```python
from build123d import *

# Parameters (mm, degrees)
F0_R     = 3.5687
F0_R_2   = 25.4
F1_DEPTH = 12.7
F2_R     = 25.39999
F3_R     = 19.05
F4_R     = 6.35


# Not quite as in the source:
# - a fillet or chamfer is up to 0.001 mm smaller than in the source, because OpenCascade refuses the exact size


with BuildPart() as f1:
    # F0 (on Top) → F1 (new body)
    with BuildSketch(Plane.XY):
        with BuildLine():
            Line((-25.4, -44.45), (0, -44.45))
            ThreePointArc((0, -44.45), (44.45, 0), (0, 44.45))
            Line((0, 44.45), (-25.4, 44.45))
            Line((-25.4, 44.45), (-25.4, 209.55))
            Line((-25.4, 209.55), (-138.1252, 322.2752))
            Line((-138.1252, 322.2752), (-352.425, 322.2752))
            Line((-352.425, 322.2752), (-352.425, 315.9252107143))
            Line((-352.425, 315.9252107143), (-387.35, 315.9252107143))
            Line((-387.35, 315.9252107143), (-387.35, 322.2752))
            Line((-387.35, 322.2752), (-584.2, 322.2752))
            Line((-584.2, 322.2752), (-584.2, 246.0752))
            Line((-584.2, 246.0752), (-187.648785695, 246.0752))
            Line((-187.648785695, 246.0752), (-114.3, 172.726414305))
            Line((-114.3, 172.726414305), (-114.3, -172.726414305))
            Line((-114.3, -172.726414305), (-200.348785695, -258.7752))
            Line((-200.348785695, -258.7752), (-400.05, -258.7752))
            Line((-400.05, -258.7752), (-400.05, -322.2752))
            Line((-400.05, -322.2752), (-138.1252, -322.2752))
            Line((-138.1252, -322.2752), (-25.4, -209.55))
            Line((-25.4, -209.55), (-25.4, -44.45))
        make_face()
        with Locations((-385.3688, -303.2252)):
            Circle(F0_R, mode=Mode.SUBTRACT)
        with Locations((-350.4438, -303.2252)):
            Circle(F0_R, mode=Mode.SUBTRACT)
        with Locations((-385.3688, -277.8252)):
            Circle(F0_R, mode=Mode.SUBTRACT)
        with Locations((-350.4438, -277.8252)):
            Circle(F0_R, mode=Mode.SUBTRACT)
        with BuildLine():
            Line((-503.2502, 258.3815), (-563.5752, 258.3815))
            ThreePointArc((-563.5752, 258.3815), (-567.1439, 261.9502), (-563.5752, 265.5189))
            Line((-563.5752, 265.5189), (-503.2502, 265.5189))
            ThreePointArc((-503.2502, 265.5189), (-499.6815, 261.9502), (-503.2502, 258.3815))
        make_face(mode=Mode.SUBTRACT)
        with BuildLine():
            ThreePointArc((-563.5752, 283.7815), (-567.1439, 287.3502), (-563.5752, 290.9189))
            Line((-563.5752, 290.9189), (-503.2502, 290.9189))
            ThreePointArc((-503.2502, 290.9189), (-499.6815, 287.3502), (-503.2502, 283.7815))
            Line((-503.2502, 283.7815), (-563.5752, 283.7815))
        make_face(mode=Mode.SUBTRACT)
        with BuildLine():
            Line((-282.575, 264.7315), (-314.325, 264.7315))
            ThreePointArc((-314.325, 264.7315), (-317.8937, 268.3002), (-314.325, 271.8689))
            Line((-314.325, 271.8689), (-282.575, 271.8689))
            ThreePointArc((-282.575, 271.8689), (-279.0063, 268.3002), (-282.575, 264.7315))
        make_face(mode=Mode.SUBTRACT)
        with BuildLine():
            Line((-282.575, 290.1315), (-314.325, 290.1315))
            ThreePointArc((-314.325, 290.1315), (-317.8937, 293.7002), (-314.325, 297.2689))
            Line((-314.325, 297.2689), (-282.575, 297.2689))
            ThreePointArc((-282.575, 297.2689), (-279.0063, 293.7002), (-282.575, 290.1315))
        make_face(mode=Mode.SUBTRACT)
        Circle(F0_R_2, mode=Mode.SUBTRACT)
        with BuildLine():
            Line((-190.5, 258.3815), (-250.825, 258.3815))
            ThreePointArc((-250.825, 258.3815), (-254.3937, 261.9502), (-250.825, 265.5189))
            Line((-250.825, 265.5189), (-190.5, 265.5189))
            ThreePointArc((-190.5, 265.5189), (-186.9313, 261.9502), (-190.5, 258.3815))
        make_face(mode=Mode.SUBTRACT)
        with BuildLine():
            ThreePointArc((-250.825, 283.7815), (-254.3937, 287.3502), (-250.825, 290.9189))
            Line((-250.825, 290.9189), (-190.5, 290.9189))
            ThreePointArc((-190.5, 290.9189), (-186.9313, 287.3502), (-190.5, 283.7815))
            Line((-190.5, 283.7815), (-250.825, 283.7815))
        make_face(mode=Mode.SUBTRACT)
    extrude(amount=F1_DEPTH)

    # F2 (radius 25.4 in the source; OpenCascade refuses exactly that, so slightly less here)
    f2_edges = [f1.edges().sort_by_distance(p)[0] for p in [
        (-25.4, -44.45, 6.35),
        (-25.4, 44.45, 6.35),
    ]]
    fillet(f2_edges, radius=F2_R)

    # F3
    f3_edges = [f1.edges().sort_by_distance(p)[0] for p in [
        (-25.4, -209.55, 6.35),
        (-138.1252, -322.2752, 6.35),
        (-25.4, 209.55, 6.35),
        (-138.1252, 322.2752, 6.35),
        (-114.3, 172.726414, 6.35),
        (-187.648786, 246.0752, 6.35),
        (-114.3, -172.726414, 6.35),
        (-200.348786, -258.7752, 6.35),
    ]]
    fillet(f3_edges, radius=F3_R)

    # F4
    f4_edges = [f1.edges().sort_by_distance(p)[0] for p in [
        (-400.05, -258.7752, 6.35),
        (-400.05, -322.2752, 6.35),
        (-584.2, 246.0752, 6.35),
        (-584.2, 322.2752, 6.35),
    ]]
    fillet(f4_edges, radius=F4_R)


solid = f1.part
```
Read the model definition and answer for the solid it produces. Units are mm, in the model's axes. A direction names the side the tool comes from. Give positions to 0.01 mm unless a question says otherwise; leave off trailing zeros. Order: outer loops, then holes, each group sorted by start corner. A loop starts at its lowest first (then second) coordinate and runs counter-clockwise, first axis right, second up.
(1) For faces 1 (the flat face through (-151.41, 209.836, 6.261)), 2 (the cylindrical face through (-5.506, -24.796, 6.261)), determine the directions among +Z, -Z, +X, -X, +Y, -Y from which every point of the face is accessible in a straight line to the end or side of a thin tool.
(2) Find section C-C (x = -369.5). Give the vertices of the cut face in (y, z).
(3) For a pull along Y with two mould halves and no side action, classify faces 3 (the flat face through (-81.05, 265.2, 6.26)), 4 (the cylindrical face through (-17.76, -51.69, 6.44)), 5 (the flat face through (-156.8, -215.227, 6.261)) as released by +Y, released by -Y, zero draft, split by the parting line, or undercut.
(4) Find section A-A (x = -235). Give the vertices of the cut face in (y, z), plus the area to 3 significant figures.
(5) Straight lines are drawn through the part: L1, parallel to Y at x = -535.5, z = 9.75; L2, parallel to Y at x = -212.5, z = 1.5; L3, parallel to Y at x = -289, z = 4.25. For each, find the intervals that lie inside material, in ascending order.
(6) Find section D-D (x = -92). Give the vertices of the cut face in (y, z).
(7) Find section B-B (y = 0). Give the vertices of the cut face in (x, z), plus the area to 3 significant figures.
(8) Given pin 1 (4 mm diameter, centred on y = -148, z = 8, fed in from +X); pin 2 (1.5 mm diameter, centred on y = 202, z = 10.5, fed in from -X); pin 3 (6 mm diameter, centred on x = -30, z = 8, fed in from +Y), each flat-ended and moving along its own axis, determine where each tip first touches the part or whether it passes through.
Result sheet:
1. face 1: +Z, -Z, -X
1. face 2: +Z, -Z
2. outline: (-322.28, 0) - (-258.78, 0) - (-258.78, 12.7) - (-322.28, 12.7) - close; (246.08, 0) - (315.93, 0) - (315.93, 12.7) - (246.08, 12.7) - close
3. face 3: released by +Y
3. face 4: released by -Y
3. face 5: undercut
4. outline: (-322.28, 0) - (-258.78, 0) - (-258.78, 12.7) - (-322.28, 12.7) - close; (246.08, 0) - (258.38, 0) - (258.38, 12.7) - (246.08, 12.7) - close; (265.52, 0) - (283.78, 0) - (283.78, 12.7) - (265.52, 12.7) - close; (290.92, 0) - (322.28, 0) - (322.28, 12.7) - (290.92, 12.7) - close
4. area: 1,590 mm2
5. L1: y = 246.08 to 258.38, 265.52 to 283.78, 290.92 to 322.28
5. L2: y = -322.28 to -258.78, 246.08 to 258.38, 265.52 to 283.78, 290.92 to 322.28
5. L3: y = -322.28 to -258.78, 246.08 to 264.73, 271.87 to 290.13, 297.27 to 322.28
6. outline: (-276.15, 0) - (276.15, 0) - (276.15, 12.7) - (-276.15, 12.7) - close
7. outline: (-114.3, 0) - (-25.4, 0) - (-25.4, 12.7) - (-114.3, 12.7) - close; (25.4, 0) - (44.45, 0) - (44.45, 12.7) - (25.4, 12.7) - close
7. area: 1,370 mm2
8. pin 1: stops at x = -25.4
8. pin 2: stops at x = -144.32
8. pin 3: stops at y = 217.15
